Verification items for the finished model (mm, model axes). Face numbers are marked on the shaded views. A direction names the side the tool comes from. Give positions to 0.01 mm unless a question says otherwise; leave off trailing zeros. Loops run counter-clockwise (first coordinate to the right, second up) from the corner with the lowest first, then second, coordinate; pieces in that order, holes last. Notation, with made-up numbers: (78.25, 44.5) - (90.25, 44.5) arc R28 ccw to (90.25, 75.5) - close; hole circle Ø8 at (63, 73.5). An arc over 180 degrees is marked (long way). Answer in a Markdown table with one row per item.
```python
from build123d import *

# Parameters (mm, degrees)
SKETCH2_W           = 140.5
SKETCH2_H           = 98.5
BOSS_EXTRUDE6_DEPTH = 10
SKETCH10_W          = 100.6
SKETCH10_H          = 71
CUT_EXTRUDE4_DEPTH  = 172.8793181275746
CUT_EXTRUDE1_DEPTH  = 172.8793181275746
SKETCH5_W           = 100.6
SKETCH5_H           = 6
BOSS_EXTRUDE3_DEPTH = 2
CUT_EXTRUDE2_DEPTH  = 172.8793181275746
SKETCH4_4_R         = 1.5999999999999908
SKETCH4_4_R_2       = 1.599999999999993
SKETCH4_4_R_3       = 1.6000000000000039
SKETCH4_4_R_4       = 1.6000000000000003
BOSS_EXTRUDE7_DEPTH = 10
FILLET1_R           = 3
SKETCH4_3_R         = 1.5999999999999908
SKETCH4_3_R_2       = 1.599999999999993
SKETCH4_3_R_3       = 1.6000000000000039
SKETCH4_3_R_4       = 1.6000000000000003
BOSS_EXTRUDE2_DEPTH = 10
SKETCH7_W           = 100.6
SKETCH7_H           = 27.5
CUT_EXTRUDE3_DEPTH  = 8
SKETCH8_W           = 15.000000000000007
SKETCH8_H           = 25.5
BOSS_EXTRUDE4_DEPTH = 5.8
BOSS_EXTRUDE5_DEPTH = 4
FILLET2_R           = 3


with BuildPart() as part:
    # Sketch2 → Boss-Extrude6 (new body)
    with BuildSketch(Plane.XY):
        with Locations((70.25, 49.25)):
            Rectangle(SKETCH2_W, SKETCH2_H)
    extrude(amount=BOSS_EXTRUDE6_DEPTH)

    # Sketch10 → Cut-Extrude4 (cut, through all)
    with BuildSketch(Plane(origin=(0, 0, 0), x_dir=(-1, 0, 0), z_dir=(0, 0, -1))):
        with Locations((-70.25000000000001, 35.5)):
            Rectangle(SKETCH10_W, SKETCH10_H)
    extrude(amount=-CUT_EXTRUDE4_DEPTH, mode=Mode.SUBTRACT)

    # Sketch3 → Cut-Extrude1 (cut, through all)
    with BuildSketch(Plane.XZ):
        Polygon((17.950000000000006, 7.800000000000001), (122.55000000000001, 7.800000000000013), (122.55000000000001, 6.000000000000013), (17.950000000000006, 6), align=None)
    extrude(amount=-CUT_EXTRUDE1_DEPTH, mode=Mode.SUBTRACT)

    # Sketch5 → Boss-Extrude3 (add)
    with BuildSketch(Plane.XY):
        with Locations((70.25000000000001, 3)):
            Rectangle(SKETCH5_W, SKETCH5_H)
        Polygon((21.57809178761083, 3.480214864097709), (122.17809178761084, 68.48021486409772), (118.92190821238917, 73.51978513590232), (18.321908212389175, 8.519785135902309), align=None)
        Polygon((18.32190821238918, 68.48021486409769), (118.92190821238916, 3.4802148640977055), (122.17809178761082, 8.519785135902305), (21.578091787610838, 73.5197851359023), align=None)
    extrude(amount=BOSS_EXTRUDE3_DEPTH)

    # Sketch4 → Cut-Extrude2 (cut, through all)
    with BuildSketch(Plane.XY):
        with BuildLine():
            ThreePointArc((120.05000000000001, 4.44e-15), (121.50773797371134, 0.46899039884100846), (122.41854385646542, 1.6999999999999988))
            Line((122.41854385646542, 1.7000000000000002), (123.05000000000001, 1.7000000000000002))
            ThreePointArc((123.05000000000001, 1.7000000000000028), (123.75710678118656, 1.99289321881345), (124.05000000000001, 2.7))
            Line((124.05000000000001, 2.7), (124.05000000000001, 12.999999999999996))
            Line((124.05000000000001, 12.999999999999998), (123.25000000000001, 12.999999999999998))
            Line((123.25000000000001, 12.999999999999998), (123.25000000000001, 2.5))
            Line((123.25000000000001, 2.5), (117.55, 2.5))
            Line((117.55, 2.5), (117.55, 0))
            Line((117.55, 0), (118.55, 0))
            Line((118.55, 0), (120.05000000000001, 0))
        make_face()
        with BuildLine():
            ThreePointArc((144.50000000000003, 2), (145.20710678118658, 2.2928932188134525), (145.50000000000006, 3))
            Line((145.50000000000006, 3), (145.50000000000003, -0.5000000000000178))
            Line((145.50000000000003, -0.5000000000000178), (127.05, -0.5000000000000178))
            Line((127.05, -0.5000000000000178), (126.85, -0.5000000000000178))
            ThreePointArc((126.85, -0.5000000000000178), (125.4357864376269, 0.08578643762688709), (124.85, 1.499999999999982))
            Line((124.85, 1.499999999999982), (124.85, 12))
            ThreePointArc((124.85, 12), (125.14289321881344, 12.707106781186548), (125.85, 12.999999999999998))
            Line((125.85, 12.999999999999998), (126.35, 13))
            ThreePointArc((126.35, 13), (126.70355339059327, 12.853553390593271), (126.85, 12.499999999999998))
            Line((126.85, 12.499999999999998), (126.85, 4))
            ThreePointArc((126.85, 4), (127.4357864376269, 2.585786437626905), (128.85, 2))
            Line((128.85, 2), (144.50000000000003, 2))
        make_face()
    extrude(amount=CUT_EXTRUDE2_DEPTH, mode=Mode.SUBTRACT)

    # Sketch4<4> → Boss-Extrude7 (add, through all)
    # profile 1 of 4: a face of its own
    with BuildSketch(Plane.XY):
        with BuildLine():
            Line((128.85, 2), (144.50000000000003, 2))
            ThreePointArc((144.50000000000003, 2), (145.20710678118658, 2.2928932188134525), (145.50000000000006, 3))
            Line((145.50000000000006, 3), (145.50000000000003, 22.5))
            Line((145.50000000000003, 22.5), (140.5, 22.500000000000004))
            Line((140.5, 22.500000000000004), (124.05000000000001, 22.5))
            Line((124.05000000000001, 22.5), (124.05000000000001, 12.999999999999998))
            Line((124.05000000000001, 12.999999999999998), (124.05000000000001, 2.7))
            ThreePointArc((124.05000000000001, 2.7), (123.75710678118656, 1.9928932188134527), (123.05000000000001, 1.7000000000000002))
            Line((123.05000000000001, 1.7000000000000002), (122.41854385646542, 1.7000000000000002))
            ThreePointArc((122.41854385646542, 1.7000000000000002), (121.50773797371134, 0.4689903988410107), (120.05000000000001, 0))
            Line((120.05000000000001, 0), (118.55, 0))
            Line((118.55, 0), (118.55, -1.2))
            Line((118.55, -1.2), (122.05, -2.409773966310486))
            Line((122.05, -2.409773966310486), (123.05, -8.50000000000002))
            Line((123.05, -8.50000000000002), (127.05, -8.500000000000018))
            Line((127.05, -8.500000000000018), (127.05, -0.5000000000000178))
            Line((127.05, -0.5000000000000178), (126.85, -0.5000000000000178))
            ThreePointArc((126.85, -0.5000000000000178), (125.4357864376269, 0.08578643762688709), (124.85, 1.499999999999982))
            Line((124.85, 1.499999999999982), (124.85, 12))
            ThreePointArc((124.85, 12), (125.14289321881344, 12.707106781186548), (125.85, 12.999999999999998))
            Line((125.85, 12.999999999999998), (126.35, 13))
            ThreePointArc((126.35, 13), (126.70355339059327, 12.853553390593271), (126.85, 12.499999999999998))
            Line((126.85, 12.499999999999998), (126.85, 4))
            ThreePointArc((126.85, 4), (127.4357864376269, 2.585786437626905), (128.85, 2))
        make_face()
        with Locations((142.50000000000003, 17.5)):
            Circle(SKETCH4_4_R, mode=Mode.SUBTRACT)
    # profile 2 of 4: a face of its own
    with BuildSketch(Plane.XY):
        Polygon((145.50000000000003, 98.5), (145.50000000000003, 86.50000000000001), (140.5, 86.50000000000003), (140.5, 98.5), align=None)
        with Locations((142.5, 92.5)):
            Circle(SKETCH4_4_R_2, mode=Mode.SUBTRACT)
    # profile 3 of 4: a face of its own
    with BuildSketch(Plane.XY):
        Polygon((0, 98.49999999999999), (0, 86.50000000000001), (-5.000000000000004, 86.5), (-5.000000000000004, 98.49999999999999), align=None)
        with Locations((-1.9999999999999913, 92.5)):
            Circle(SKETCH4_4_R_3, mode=Mode.SUBTRACT)
    # profile 4 of 4: a face of its own
    with BuildSketch(Plane.XY):
        Polygon((8.67e-15, 22.499999999999986), (1.041e-14, 10.49999999999999), (-4.999999999999993, 10.499999999999986), (-4.999999999999996, 22.499999999999982), align=None)
        with Locations((-2.0000000000000018, 17.5)):
            Circle(SKETCH4_4_R_4, mode=Mode.SUBTRACT)
    extrude(amount=BOSS_EXTRUDE7_DEPTH)

    # Fillet1
    fillet1_edges = [part.edges().sort_by_distance(p)[0] for p in [
        (19.95000000000001, 67.42826688999527, 1),
        (19.949999999999992, 9.571733110004725, 1),
        (25.4779438594842, 71.00000000000001, 1),
        (115.02205614051576, 71, 1),
        (120.55000000000001, 9.571733110004711, 1),
        (120.55000000000003, 67.42826688999531, 1),
        (75.77794385948422, 38.50000000000003, 1),
        (70.24999999999997, 42.07173311000473, 1),
        (64.72205614051575, 38.499999999999986, 1),
        (25.477943859484185, 6.000000000000001, 1),
        (70.25, 34.928266889995285, 1),
        (115.0220561405158, 5.999999999999968, 1),
    ]]
    fillet(fillet1_edges, radius=FILLET1_R)

    # Sketch4<3> → Boss-Extrude2 (add, through all)
    # profile 1 of 4: a face of its own
    with BuildSketch(Plane.XY):
        with BuildLine():
            Line((123.05000000000001, 1.7000000000000002), (122.41854385646542, 1.7000000000000002))
            ThreePointArc((122.41854385646542, 1.6999999999999988), (121.50773797371134, 0.46899039884100846), (120.05000000000001, 4.44e-15))
            Line((120.05000000000001, 0), (118.55, 0))
            Line((118.55, 0), (118.55, -1.2))
            Line((118.55, -1.2), (122.05, -2.409773966310486))
            Line((122.05, -2.4097739663104853), (123.05, -8.50000000000002))
            Line((123.05, -8.50000000000002), (127.05, -8.500000000000018))
            Line((127.05, -8.500000000000018), (127.05, -0.5000000000000178))
            Line((127.05, -0.5000000000000178), (126.85, -0.5000000000000178))
            ThreePointArc((126.85, -0.5000000000000151), (125.4357864376269, 0.08578643762688865), (124.85, 1.499999999999982))
            Line((124.85, 1.4999999999999822), (124.85, 12))
            ThreePointArc((124.85, 12), (125.14289321881344, 12.70710678118655), (125.85, 12.999999999999996))
            Line((125.85, 12.999999999999998), (126.35, 13))
            ThreePointArc((126.35, 13), (126.70355339059327, 12.853553390593273), (126.85, 12.499999999999998))
            Line((126.85, 12.499999999999998), (126.85, 4))
            ThreePointArc((126.85, 4), (127.4357864376269, 2.585786437626907), (128.85, 2.000000000000003))
            Line((128.85, 2), (144.50000000000003, 2))
            ThreePointArc((144.50000000000003, 2.000000000000009), (145.20710678118658, 2.292893218813456), (145.50000000000006, 3))
            Line((145.50000000000006, 3), (145.50000000000003, 22.5))
            Line((145.50000000000003, 22.5), (140.5, 22.500000000000004))
            Line((140.5, 22.500000000000004), (124.05000000000001, 22.5))
            Line((124.05000000000001, 22.5), (124.05000000000001, 12.999999999999998))
            Line((124.05000000000001, 12.999999999999996), (124.05000000000001, 2.7))
            ThreePointArc((124.05000000000001, 2.7), (123.75710678118656, 1.99289321881345), (123.05000000000001, 1.7000000000000028))
        make_face()
        with Locations((142.50000000000003, 17.5)):
            Circle(SKETCH4_3_R, mode=Mode.SUBTRACT)
    # profile 2 of 4: a face of its own
    with BuildSketch(Plane.XY):
        Polygon((145.50000000000003, 98.5), (145.50000000000003, 86.50000000000001), (140.5, 86.50000000000003), (140.5, 98.5), align=None)
        with Locations((142.5, 92.5)):
            Circle(SKETCH4_3_R_2, mode=Mode.SUBTRACT)
    # profile 3 of 4: a face of its own
    with BuildSketch(Plane.XY):
        Polygon((0, 98.49999999999999), (0, 86.50000000000001), (-5.000000000000004, 86.5), (-5.000000000000004, 98.49999999999999), align=None)
        with Locations((-1.9999999999999913, 92.5)):
            Circle(SKETCH4_3_R_3, mode=Mode.SUBTRACT)
    # profile 4 of 4: a face of its own
    with BuildSketch(Plane.XY):
        Polygon((8.67e-15, 22.499999999999986), (1.041e-14, 10.49999999999999), (-4.999999999999993, 10.499999999999986), (-4.999999999999996, 22.499999999999982), align=None)
        with Locations((-2.0000000000000018, 17.5)):
            Circle(SKETCH4_3_R_4, mode=Mode.SUBTRACT)
    extrude(amount=BOSS_EXTRUDE2_DEPTH)

    # Sketch7 → Cut-Extrude3 (cut)
    with BuildSketch(Plane.XY.offset(10)):
        with Locations((70.25000000000001, 84.75)):
            Rectangle(SKETCH7_W, SKETCH7_H)
    extrude(amount=-CUT_EXTRUDE3_DEPTH, mode=Mode.SUBTRACT)

    # Sketch8 → Boss-Extrude4 (add)
    with BuildSketch(Plane.XY.offset(2)):
        with Locations((70.25000000000001, 85.75)):
            Rectangle(SKETCH8_W, SKETCH8_H)
    extrude(amount=BOSS_EXTRUDE4_DEPTH)

    # Sketch9 → Boss-Extrude5 (add)
    with BuildSketch(Plane.XY.offset(2)):
        with BuildLine():
            ThreePointArc((120.55000000000001, 15.081836001321573), (119.67132034355964, 12.960515657761938), (117.55000000000001, 12.081836001321571))
            Line((117.55000000000001, 12.081836001321573), (117.55000000000001, 2.5))
            Line((117.55000000000001, 2.5000000000000004), (120.55000000000001, 2.5))
            Line((120.55000000000001, 2.5), (120.55000000000001, 15.081836001321573))
        make_face()
        with BuildLine():
            Line((19.95000000000001, 15.081836001321587), (19.95000000000001, 0))
            Line((19.95000000000001, 0), (22.95000000000001, 0))
            Line((22.95000000000001, 0), (22.95000000000001, 12.08183600132159))
            ThreePointArc((22.95000000000001, 12.081836001321593), (20.828679656440368, 12.960515657761945), (19.95000000000001, 15.081836001321587))
        make_face()
    extrude(amount=BOSS_EXTRUDE5_DEPTH)

    # Fillet2
    fillet2_edges = [part.edges().sort_by_distance(p)[0] for p in [
        (22.95000000000001, 12.08183600132159, 4),
        (117.55000000000001, 12.08183600132157, 4),
    ]]
    fillet(fillet2_edges, radius=FILLET2_R)


solid = part.part
```
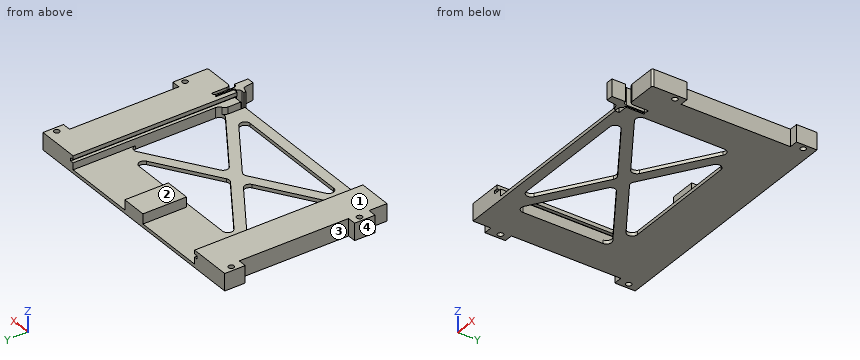
Q1. Sectioned sample at B-B (x = 142.5). Record the cut outline in (y, z), and give its area (3 significant figures).
Completed:
| item | result |
|---|---|
| outline | (2, 0) - (15.9, 0) - (15.9, 10) - (2, 10) - close; (19.1, 0) - (22.5, 0) - (22.5, 10) - (19.1, 10) - close; (86.5, 0) - (90.9, 0) - (90.9, 10) - (86.5, 10) - close; (94.1, 0) - (98.5, 0) - (98.5, 10) - (94.1, 10) - close |
| area | 261 mm^2 |
Q2. Sectioned sample at C-C (x = 112.5). Record the cut outline in (y, z), and give its area (3 significant figures).
Completed:
| item | result |
|---|---|
| outline | (0, 0) - (14.77, 0) - (14.77, 2) - (0, 2) - close; (62.23, 0) - (98.5, 0) - (98.5, 2) - (62.23, 2) - close |
| area | 102 mm^2 |
Q3. Thickness scan on line 1 (X direction, y = 87, z = 3); line 2 (X direction, y = 6, z = 6.25); line 3 (Y direction, x = 142.5, z = 6.25). Record the ranges inside material, lowest first.
Completed:
| item | result |
|---|---|
| line 1 | -5 to 19.95, 62.75 to 77.75, 120.55 to 145.5 |
| line 2 | 0 to 17.95, 122.55 to 123.25, 124.05 to 124.85, 126.85 to 145.5 |
| line 3 | 2 to 15.9, 19.1 to 22.5, 86.5 to 90.9, 94.1 to 98.5 |
Q4. Tool access check on the marked faces 1 and 2. Record the directions out of +Z, -Z, +X, -X, +Y, -Y that give a thin tool (end or side, any length) a straight path to the whole face; none if there is none.
Completed:
| item | result |
|---|---|
| face 1 | +Z, +X, -X, +Y, -Y |
| face 2 | +Z, +Y, -Y |
Q5. Draft check along Y on the marked faces 3 and 4. Enter one of: +Y half, -Y half, draft (parallel to the pull), parting line (faces both ways), or undercut.
Completed:
| item | result |
|---|---|
| face 3 | undercut |
| face 4 | draft |
Q6. Sectioned sample at A-A (y = 92.5). Record the cut outline in (x, z).
Completed:
| item | result |
|---|---|
| outline | (-5, 0) - (-3.6, 0) - (-3.6, 10) - (-5, 10) - close; (-0.4, 0) - (140.9, 0) - (140.9, 10) - (120.55, 10) - (120.55, 7.8) - (122.55, 7.8) - (122.55, 6) - (120.55, 6) - (120.55, 2) - (77.75, 2) - (77.75, 7.8) - (62.75, 7.8) - (62.75, 2) - (19.95, 2) - (19.95, 6) - (17.95, 6) - (17.95, 7.8) - (19.95, 7.8) - (19.95, 10) - (-0.4, 10) - close; (144.1, 0) - (145.5, 0) - (145.5, 10) - (144.1, 10) - close |
Q7. Sectioned sample at D-D (x = -2). Record the cut outline in (y, z).
Completed:
| item | result |
|---|---|
| outline | (10.5, 0) - (15.9, 0) - (15.9, 10) - (10.5, 10) - close; (19.1, 0) - (22.5, 0) - (22.5, 10) - (19.1, 10) - close; (86.5, 0) - (90.9, 0) - (90.9, 10) - (86.5, 10) - close; (94.1, 0) - (98.5, 0) - (98.5, 10) - (94.1, 10) - close |
Q8. Go/stop test with flat-tipped pins: P1, Ø1.2, axis at y = 6.5, z = 4, coming from the -X side; P2, Ø4.5, axis at x = 67, y = 90, coming from the +Z side; P3, Ø4, axis at x = -3.5, z = 6, coming from the -Y side. Record where each tip stops, or that it passes through.
Completed:
| item | result |
|---|---|
| P1 | x = 0 |
| P2 | z = 7.8 |
| P3 | y = 10.5 |
